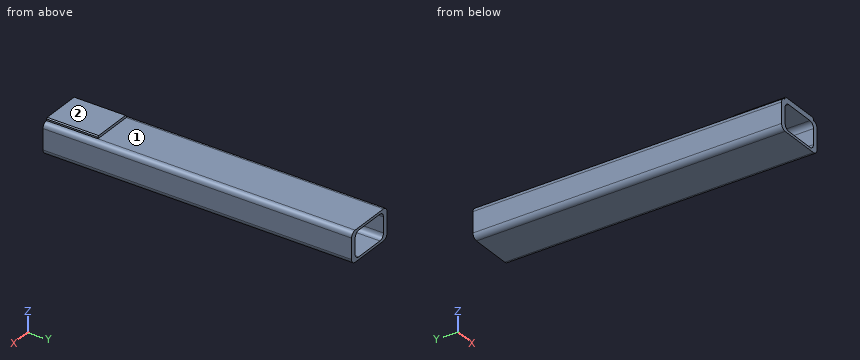
```python
from build123d import *

# Parameters (mm, degrees)
F1_DEPTH = 762
F2_W     = 101.6
F2_H     = 127
F3_DEPTH = 6.35
F4_SIZE  = 2.54


with BuildPart() as f1:
    # F0 (on Front) → F1 (new body)
    with BuildSketch(Plane.XZ):
        with BuildLine():
            ThreePointArc((63.5, 25.4), (59.780256, 34.380256), (50.8, 38.1))
            Line((50.8, 38.1), (-50.8, 38.1))
            ThreePointArc((-50.8, 38.1), (-59.780256, 34.380256), (-63.5, 25.4))
            Line((-63.5, 25.4), (-63.5, -25.4))
            ThreePointArc((-63.5, -25.4), (-59.780256, -34.380256), (-50.8, -38.1))
            Line((-50.8, -38.1), (50.8, -38.1))
            ThreePointArc((50.8, -38.1), (59.780256, -34.380256), (63.5, -25.4))
            Line((63.5, -25.4), (63.5, 25.4))
        make_face()
        with BuildLine():
            Line((-38.1, 31.75), (38.1, 31.75))
            ThreePointArc((38.1, 31.75), (47.080256, 28.030256), (50.8, 19.05))
            Line((50.8, 19.05), (50.8, -19.05))
            ThreePointArc((50.8, -19.05), (47.080256, -28.030256), (38.1, -31.75))
            Line((38.1, -31.75), (-38.1, -31.75))
            ThreePointArc((-38.1, -31.75), (-47.080256, -28.030256), (-50.8, -19.05))
            Line((-50.8, -19.05), (-50.8, 19.05))
            ThreePointArc((-50.8, 19.05), (-47.080256, 28.030256), (-38.1, 31.75))
        make_face(mode=Mode.SUBTRACT)
    extrude(amount=F1_DEPTH)

    # F2 (on face) → F3 (join)
    with BuildSketch(Plane.XY.offset(38.1)):
        with Locations((0, -698.5)):
            Rectangle(F2_W, F2_H)
    extrude(amount=F3_DEPTH)

    # F4
    f4_edges = [f1.edges().sort_by_distance(p)[0] for p in [
        (50.8, -698.5, 44.45),
        (-50.8, -698.5, 44.45),
    ]]
    chamfer(f4_edges, length=F4_SIZE)


solid = f1.part
```
Check sheet for the modelled part. Datum: model origin and axes. Units: mm. Face numbers are marked on the shaded views. A direction names the side the tool comes from. Round coordinates to 2 decimals unless told otherwise and drop trailing zeros. Loops run counter-clockwise (first coordinate to the right, second up) from the corner with the lowest first, then second, coordinate; pieces in that order, holes last. Notation, with made-up numbers: (-9, 28.25) - (40, 28.25) arc R21 cw to (40, 38.25) - close; hole circle Ø6 at (79, -31). An arc over 180 degrees is marked (long way). Answer as a JSON object with one key per item and string values. Group by question number.
Q1. Gauge pin test, flat ends, axial feed: P1, Ø6, axis at x = -16, y = -454, coming from the +Z side; P2, Ø3, axis at y = -701.5, z = 40, coming from the +X side; P3, Ø3, axis at x = -13.5, z = 41.5, coming from the +Y side. Record the tip position at first contact, or that the pin passes through.
Q2. Set-up check for the marked faces 1 and 2: record each of +Z, -Z, +X, -X, +Y, -Y from which the full face is reachable in a straight line by a thin tool's end or side.
Q3. Sectioned sample at A-A, the plane z = -5.5. Enter the section's corners in (x, y).
Q4. Sectioned sample at C-C, the plane y = -233. Enter the section's corners in (x, z).
Q5. Scan lines: line 1 along X through (y, z) = (-272.5, -8.5); line 2 along Z through (x, y) = (-9.5, -652); line 3 along Z through (x, y) = (-13, -546). Record each from-to range of solid material in increasing order. Write a range as [from, to].
Q6. Sectioned sample at B-B, the plane x = -27. Enter the section's corners in (y, z).
Solution:
{
 "1": {"P1": "stops at z = 38.1", "P2": "stops at x = 50.8", "P3": "stops at y = -635"},
 "2": {"face 1": "+Z, +X, -X, +Y", "face 2": "+Z, +X, -X, +Y, -Y"},
 "3": {"outline": "(-63.5, -762) - (-50.8, -762) - (-50.8, 0) - (-63.5, 0) - close; (50.8, -762) - (63.5, -762) - (63.5, 0) - (50.8, 0) - close"},
 "4": {"outline": "(-63.5, -25.4) arc R12.7 ccw to (-50.8, -38.1) - (50.8, -38.1) arc R12.7 ccw to (63.5, -25.4) - (63.5, 25.4) arc R12.7 ccw to (50.8, 38.1) - (-50.8, 38.1) arc R12.7 ccw to (-63.5, 25.4) - close; hole (-50.8, -19.05) arc R12.7 ccw to (-38.1, -31.75) - (38.1, -31.75) arc R12.7 ccw to (50.8, -19.05) - (50.8, 19.05) arc R12.7 ccw to (38.1, 31.75) - (-38.1, 31.75) arc R12.7 ccw to (-50.8, 19.05) - close"},
 "5": {"line 1": "x = [-63.5, -50.8], [50.8, 63.5]", "line 2": "z = [-38.1, -31.75], [31.75, 44.45]", "line 3": "z = [-38.1, -31.75], [31.75, 38.1]"},
 "6": {"outline": "(-762, -38.1) - (0, -38.1) - (0, -31.75) - (-762, -31.75) - close; (-762, 31.75) - (0, 31.75) - (0, 38.1) - (-635, 38.1) - (-635, 44.45) - (-762, 44.45) - close"}
}
